Here's how the part is built. I have some questions about the finished solid (model axes, mm). A direction names the side the tool comes from. Round coordinates to 2 decimals unless told otherwise and drop trailing zeros. Order: outer loops, then holes, each group sorted by start corner. A loop starts at its lowest first (then second) coordinate and runs counter-clockwise, first axis right, second up. Notation, with made-up numbers: (43.5, 84.25) -> (52.5, 84.25) arc R33 ccw to (52.5, 122.25) -> close; hole circle Ø10 at (37.25, 31). An arc over 180 degrees is marked (long way). Answer in a Markdown table with one row per item.
Autodesk Inventor part; units mm, degrees
ref_plane "YZ Plane" through (0, 0, 0) normal (1, 0, 0) x (0, 1, 0)
ref_plane "XZ Plane" through (0, 0, 0) normal (0, 1, 0) x (-1, 0, 0)
ref_plane "XY Plane" through (0, 0, 0) normal (0, 0, 1) x (1, 0, 0)
sketch "Цилиндр" plane through (0, 0, 0) normal (1, 0, 0) x (0, 1, 0)
  line L0 (5, 0) -> (-5, 0)
  line L1 (0, 5) -> (0, -5)
  circle A0 centre (0, 0) radius 5
  dimension "d0" = 10
extrude "Выдавливание1" add sketch "Цилиндр" along normal blind 80 and the other way blind 15.61
sketch "Корпус" plane through (-15.61, 0, 0) normal (-1, 0, 0) x (0, 0, 1)
  arc A0 (5, 0) -> (-5, 0) centre (0, 0) ccw
  circle A1 centre (0, 0) radius 5
  line L0 (0, 5) -> (0, -5)
  line L1 (-5, 0) -> (5, 0)
  line L2 (-4.999794, -5) -> (5, -5)
  arc A2 (5, 0) -> (-5, 0) centre (0, 0) ccw
  line L3 (5, 0) -> (4.993827, -5)
  line L4 (-4.993645, -5) -> (-5, 0)
  line L5 (-22.603669, -4.981004) -> (-22.603669, -6.955879)
  arc A3 (0, 7) -> (-7, -0.000001) centre (0, 0) ccw
  line L6 (-22.603669, -6.955879) -> (2.271039, -6.955879)
  line L7 (22.603669, -4.981004) -> (22.603669, -6.955879)
  arc A4 (7, -0.000001) -> (0, 7) centre (0, 0) ccw
  line L8 (22.603669, -6.955879) -> (2.271039, -6.955879)
  line L9 (-6.993669, -4.981004) -> (-7, -0.000001)
  line L10 (-22.603669, -4.981004) -> (-6.993669, -4.981004)
  line L11 (7, -0.000001) -> (6.99385, -4.981004)
  line L12 (22.603669, -4.981004) -> (6.99385, -4.981004)
  dimension "d12" = 15.61
sketch "Корпус outline for Выдавливание2" plane through (-15.61, 0, 0) normal (-1, 0, 0) x (0, 0, 1)
  line L0 (-22.603669, -6.955879) -> (-22.603669, -4.981004)
  line L1 (2.271039, -6.955879) -> (-22.603669, -6.955879)
  line L2 (-22.603669, -4.981004) -> (-6.993669, -4.981004)
  line L3 (22.603669, -6.955879) -> (2.271039, -6.955879)
  line L4 (-6.993669, -4.981004) -> (-7, -0.000001)
  line L5 (22.603669, -4.981004) -> (22.603669, -6.955879)
  arc A0 (-7, -0.000001) -> (0, 7) centre (0, 0) cw
  line L6 (6.99385, -4.981004) -> (22.603669, -4.981004)
  arc A1 (0, 7) -> (7, -0.000001) centre (0, 0) cw
  line L7 (7, -0.000001) -> (6.99385, -4.981004)
  arc A2 (5, 0) -> (0, 5) centre (0, 0) ccw
  arc A3 (0, 5) -> (-5, 0) centre (0, 0) ccw
  line L8 (-5, 0) -> (-4.993645, -5)
  line L9 (-4.993645, -5) -> (0, -5)
  line L10 (0, -5) -> (4.993827, -5)
  line L11 (4.993827, -5) -> (5, 0)
extrude "Выдавливание2" add sketch "Корпус outline for Выдавливание2" against normal blind 80
sketch "Выемка" plane through (64.39, -0.000001, -7) normal (0, -0.001271, -0.9999992) x (-1, 0, 0)
  line L0 (80, -4.981007) -> (80, 0)
  line L1 (80, 0) -> (0, 0)
  line L2 (0, -4.981007) -> (0, 0)
  line L3 (80, -4.981007) -> (0, -4.981007)
  line L4 (80, -5.008896) -> (-15.61, -5.008896)
  line L5 (80, 6.991104) -> (0, 6.991104)
  line L6 (33.204769, 6.991104) -> (33.204769, -5.008896)
  line L7 (33.204769, 6.991104) -> (73.204769, 6.991104)
  line L8 (73.204769, -5.008896) -> (73.204769, 6.991104)
  line L9 (33.204769, -5.008896) -> (73.204769, -5.008896)
  line L10 (38.204769, 1.959942) -> (38.204769, -5.008896)
  line L11 (68.204769, 1.959942) -> (68.204769, -5.008896)
  line L12 (38.204769, -5.008896) -> (38.204769, 1.959942)
  line L13 (68.204769, 1.959942) -> (38.204769, 1.959942)
  line L14 (33.204769, -5.008896) -> (38.204769, -5.008896)
  line L15 (68.204769, -5.008896) -> (73.204769, -5.008896)
  point P0 (64.39, -0.008896)
  dimension "d15" = 30
  dimension "d22" = 5
  dimension "d23" = 5
extrude "Выдавливание3" cut sketch "Выемка" against normal blind 2 contours L8 L4 L11 L3 | L3 L11 L1 L8 | L1 L11 L13 L10 L6 L5 L8 | L10 L4 L6 L3 | L3 L6 L1 L10
properties part number "lw_5"
1. We'd pull the mould along X, two halves only. Please class faces 3 (the face through (24, -6.956, 0)), 4 (the face through (31.185, -1, -6)), 5 (the face through (64.39, -6, -2)), 6 (the face through (-8.815, -1, -6)): released by +X, released by -X, zero draft, split by the parting line, or undercut.
Numbers:
| item | result |
|---|---|
| face 3 | zero draft |
| face 4 | undercut |
| face 5 | released by +X |
| face 6 | undercut |
2. For pin 1 Ø1 at (x, z) = (8, 17.5) entering from +Y; pin 2 Ø17 at (x, z) = (44, -11.5) entering from +Y; pin 3 Ø1 at (y, z) = (0.5, -6) entering from +X; pin 4 Ø8 at (y, z) = (4.5, 13) entering from -X, each with a flat end and sliding along its axis, tell me the tip position at first contact or that it passes through.
Numbers:
| item | result |
|---|---|
| pin 1 | stops at y = -4.98 |
| pin 2 | stops at y = 6.32 |
| pin 3 | stops at x = 64.39 |
| pin 4 | passes through |
3. Suppose I cut it at A-A on z = -4. Write out the boundary of the cut face in (x, y), then the cut area to 3 significant figures.
Numbers:
| item | result |
|---|---|
| outline | (-15.61, -6.96) -> (64.39, -6.96) -> (64.39, -5) -> (-15.61, -5) -> close; (-15.61, -3) -> (80, -3) -> (80, 3) -> (64.39, 3) -> (64.39, 5.74) -> (-15.61, 5.74) -> close |
| area | 950 mm2 |
4. Please list where these lines run through material, in increasing order: line 1 along Y through (x, z) = (9, -10); line 2 along Z through (x, y) = (27.5, -3); line 3 along Z through (x, y) = (61, -4.25).
Numbers:
| item | result |
|---|---|
| line 1 | y = -6.96 to -4.98 |
| line 2 | z = -4 to 4, 5 to 7 |
| line 3 | z = -6.99 to -4.99, -2.63 to 2.63, 4.99 to 6.99 |
5. Suppose I cut it at B-B on y = -1.5. Write out the boundary of the cut face in (x, z).
Numbers:
| item | result |
|---|---|
| outline | (-15.61, -7) -> (-8.81, -7) -> (-8.81, -5) -> (-15.61, -5) -> close; (-15.61, -4.77) -> (80, -4.77) -> (80, 4.77) -> (-15.61, 4.77) -> close; (-15.61, 5) -> (64.39, 5) -> (64.39, 7) -> (-15.61, 7) -> close; (-3.81, -7) -> (26.19, -7) -> (26.19, -5) -> (-3.81, -5) -> close; (31.19, -7) -> (64.39, -7) -> (64.39, -5) -> (31.19, -5) -> close |
6. For faces 1 (the face through (24, -4.981, -15)), 2 (the face through (24, -6, -22.604)), which set-ups out of +Z, -Z, +X, -X, +Y, -Y let a thin tool reach every point of the face, with its end or its side?
Numbers:
| item | result |
|---|---|
| face 1 | -Z, +X, -X, +Y |
| face 2 | -Z, +X, -X, +Y, -Y |
7. Suppose I cut it at C-C on z = 10.5. Write out the boundary of the cut face in (x, y), then the cut area to 3 significant figures.
Numbers:
| item | result |
|---|---|
| outline | (-15.61, -6.96) -> (64.39, -6.96) -> (64.39, -4.98) -> (-15.61, -4.98) -> close |
| area | 158 mm2 |
